Build history of the part. All positions in model axes, mm. A direction names the side the tool comes from. Round coordinates to 2 decimals unless told otherwise and drop trailing zeros. Loops run counter-clockwise (first coordinate to the right, second up) from the corner with the lowest first, then second, coordinate; pieces in that order, holes last. Notation, with made-up numbers: M 58.25,26.25 L 83.25,26.25 A18 cw 83.25,36.25 Z; hole C 32,54.5 d5. An arc over 180 degrees is marked long. Write each question's results on one line, items separated by ' | '. Start each with the question number.
```python
from build123d import *

# Parameters (mm, degrees)
SKETCH1_W           = 30
SKETCH1_H           = 30
BOSS_EXTRUDE2_DEPTH = 15
SKETCH3_W           = 20
SKETCH3_H           = 20
CUT_EXTRUDE1_DEPTH  = 5
SKETCH4_R           = 5
CUT_EXTRUDE2_DEPTH  = 8
SKETCH7_R           = 2
CUT_EXTRUDE4_DEPTH  = 25
SKETCH8_W           = 10
SKETCH8_H           = 10
CUT_EXTRUDE7_DEPTH  = 25
SKETCH9_W           = 30
SKETCH9_H           = 8
CUT_EXTRUDE8_DEPTH  = 25
FILLET1_R           = 2
FILLET2_R           = 2


with BuildPart() as part:
    # Sketch1 → Boss-Extrude2 (new body)
    with BuildSketch(Plane(origin=(0, 0, 0), x_dir=(1, 0, 0), z_dir=(0, 1, 0))):
        with Locations((15, 15)):
            Rectangle(SKETCH1_W, SKETCH1_H)
    extrude(amount=BOSS_EXTRUDE2_DEPTH)

    # Sketch3 → Cut-Extrude1 (cut)
    with BuildSketch(Plane(origin=(0, 15, 0), x_dir=(1, 0, 0), z_dir=(0, 1, 0))):
        with Locations((15, 10)):
            Rectangle(SKETCH3_W, SKETCH3_H)
    extrude(amount=-CUT_EXTRUDE1_DEPTH, mode=Mode.SUBTRACT)

    # Sketch4 → Cut-Extrude2 (cut)
    with BuildSketch(Plane.XZ):
        with Locations(Location((15, -11, 0), (0, 0, 270))):
            Circle(SKETCH4_R)
    extrude(amount=-CUT_EXTRUDE2_DEPTH, mode=Mode.SUBTRACT)

    # Sketch7 → Cut-Extrude4 (cut)
    with BuildSketch(Plane(origin=(0, 10, 0), x_dir=(1, 0, 0), z_dir=(0, 1, 0))):
        with Locations(Location((7, 18, 0), (0, 0, 90))):
            Circle(SKETCH7_R)
        with Locations(Location((23, 18, 0), (0, 0, 90))):
            Circle(SKETCH7_R)
    extrude(amount=-CUT_EXTRUDE4_DEPTH, mode=Mode.SUBTRACT)

    # Sketch8 → Cut-Extrude7 (cut)
    with BuildSketch(Plane(origin=(0, 15, 0), x_dir=(1, 0, 0), z_dir=(0, 1, 0))):
        with Locations((15, 25)):
            Rectangle(SKETCH8_W, SKETCH8_H)
    extrude(amount=-CUT_EXTRUDE7_DEPTH, mode=Mode.SUBTRACT)

    # Sketch9 → Cut-Extrude8 (cut)
    with BuildSketch(Plane(origin=(0, 15, 0), x_dir=(1, 0, 0), z_dir=(0, 1, 0))):
        with Locations((15, 26)):
            Rectangle(SKETCH9_W, SKETCH9_H)
    extrude(amount=-CUT_EXTRUDE8_DEPTH, mode=Mode.SUBTRACT)

    # Fillet1
    # the kernel refuses this fillet: 2 mm, written as the material it takes off along each edge
    with BuildSketch(Plane(origin=(20, 0, -20), x_dir=(1, 0, 0), z_dir=(0, 0, -1)), Plane(origin=(10, 0, -27), x_dir=(-1, 0, 0), z_dir=(0, 0, 1))) as fillet1_piece_1:
        with BuildLine():
            CenterArc((FILLET1_R, -FILLET1_R), FILLET1_R, 90, 90)
            Line((0, -FILLET1_R), (0, 0))
            Line((0, 0), (FILLET1_R, 0))
        make_face()
    extrude(amount=7, mode=Mode.SUBTRACT)
    with BuildSketch(Plane(origin=(10, 0, -20), x_dir=(0, 0, 1), z_dir=(1, 0, 0))) as fillet1_piece_2:
        with BuildLine():
            CenterArc((FILLET1_R, -FILLET1_R), FILLET1_R, 90, 90)
            Line((0, -FILLET1_R), (0, 0))
            Line((0, 0), (FILLET1_R, 0))
        make_face()
    extrude(amount=10, mode=Mode.SUBTRACT)
    with BuildSketch(Plane(origin=(15, 0, -22), x_dir=(0, 0, 1), z_dir=(-1, 0, 0)), Plane(origin=(35, 0, -22), x_dir=(0, 0, 1), z_dir=(-1, 0, 0))) as fillet1_piece_3:
        with BuildLine():
            CenterArc((FILLET1_R, FILLET1_R), FILLET1_R, 180, 90)
            Line((0, FILLET1_R), (0, 0))
            Line((0, 0), (FILLET1_R, 0))
        make_face()
    extrude(amount=20, mode=Mode.SUBTRACT)
    with BuildSketch(Plane(origin=(0, 0, -27), x_dir=(1, 0, 0), z_dir=(0, 0, 1)), Plane(origin=(30, 0, 5), x_dir=(-1, 0, 0), z_dir=(0, 0, -1))) as fillet1_piece_4:
        with BuildLine():
            CenterArc((FILLET1_R, FILLET1_R), FILLET1_R, 180, 90)
            Line((0, FILLET1_R), (0, 0))
            Line((0, 0), (FILLET1_R, 0))
        make_face()
    extrude(amount=32, mode=Mode.SUBTRACT)
    with BuildSketch(Plane(origin=(-5, 0, 0), x_dir=(0, 1, 0), z_dir=(1, 0, 0))) as fillet1_piece_5:
        with BuildLine():
            CenterArc((FILLET1_R, -FILLET1_R), FILLET1_R, 90, 90)
            Line((0, -FILLET1_R), (0, 0))
            Line((0, 0), (FILLET1_R, 0))
        make_face()
    extrude(amount=40, mode=Mode.SUBTRACT)
    with BuildSketch(Plane(origin=(10, 0, -20), x_dir=(0, 0, 1), z_dir=(1, 0, 0))) as fillet1_piece_6a_section:
        with BuildLine():
            CenterArc((FILLET1_R, -FILLET1_R), FILLET1_R, 90, 90)
            Line((0, -FILLET1_R), (0, 0))
            Line((0, 0), (FILLET1_R, 0))
        make_face()
    fillet1_piece_6a = extrude(amount=15, mode=Mode.PRIVATE)
    fillet1_piece_6a = split(fillet1_piece_6a, bisect_by=Plane(origin=(20, 0.452790229, -19.547209771), z_dir=(1, 0, 0)), keep=Keep.TOP, mode=Mode.PRIVATE)
    with BuildSketch(Plane(origin=(20, 0, -15), x_dir=(1, 0, 0), z_dir=(0, 0, -1))) as fillet1_piece_6b_section:
        with BuildLine():
            CenterArc((FILLET1_R, -FILLET1_R), FILLET1_R, 90, 90)
            Line((0, -FILLET1_R), (0, 0))
            Line((0, 0), (FILLET1_R, 0))
        make_face()
    fillet1_piece_6b = extrude(amount=12, mode=Mode.PRIVATE)
    fillet1_piece_6b = split(fillet1_piece_6b, bisect_by=Plane(origin=(20.452790229, 0.452790229, -20), z_dir=(0, 0, 1)), keep=Keep.TOP, mode=Mode.PRIVATE)
    fillet1_piece_6 = fillet1_piece_6a & fillet1_piece_6b
    add(fillet1_piece_6, mode=Mode.SUBTRACT)
    with BuildSketch(Plane(origin=(10, 0, -27), x_dir=(-1, 0, 0), z_dir=(0, 0, 1))) as fillet1_piece_7a_section:
        with BuildLine():
            CenterArc((FILLET1_R, -FILLET1_R), FILLET1_R, 90, 90)
            Line((0, -FILLET1_R), (0, 0))
            Line((0, 0), (FILLET1_R, 0))
        make_face()
    fillet1_piece_7a = extrude(amount=12, mode=Mode.PRIVATE)
    fillet1_piece_7a = split(fillet1_piece_7a, bisect_by=Plane(origin=(9.547209771, 0.452790229, -20), z_dir=(0, 0, 1)), keep=Keep.TOP, mode=Mode.PRIVATE)
    with BuildSketch(Plane(origin=(5, 0, -20), x_dir=(0, 0, 1), z_dir=(1, 0, 0))) as fillet1_piece_7b_section:
        with BuildLine():
            CenterArc((FILLET1_R, -FILLET1_R), FILLET1_R, 90, 90)
            Line((0, -FILLET1_R), (0, 0))
            Line((0, 0), (FILLET1_R, 0))
        make_face()
    fillet1_piece_7b = extrude(amount=15, mode=Mode.PRIVATE)
    fillet1_piece_7b = split(fillet1_piece_7b, bisect_by=Plane(origin=(10, 0.452790229, -19.547209771), z_dir=(-1, 0, 0)), keep=Keep.TOP, mode=Mode.PRIVATE)
    fillet1_piece_7 = fillet1_piece_7a & fillet1_piece_7b
    add(fillet1_piece_7, mode=Mode.SUBTRACT)

    # Fillet2
    # the kernel refuses this fillet: 2 mm, written as the material it takes off along each edge
    with BuildSketch(Plane(origin=(2, 2, -2), x_dir=(-1, 0, 0), z_dir=(0, 0, 1))) as fillet2_piece_1_section:
        Polygon((0, 0), (FILLET2_R, 0), (FILLET2_R, FILLET2_R), (0, FILLET2_R), align=None)
    fillet2_piece_1 = extrude(amount=FILLET2_R, mode=Mode.PRIVATE)
    fillet2_piece_1 = fillet2_piece_1 - Plane(origin=(2, 2, -2), x_dir=(0.7071067811865475, 0.7071067811865475, 0), z_dir=(0, 0, 1)) * Sphere(FILLET2_R, mode=Mode.PRIVATE)
    add(fillet2_piece_1, mode=Mode.SUBTRACT)
    with BuildSketch(Plane(origin=(2, 2, -20), x_dir=(0, 0, -1), z_dir=(-1, 0, 0))) as fillet2_piece_2_section:
        Polygon((0, 0), (FILLET2_R, 0), (FILLET2_R, FILLET2_R), (0, FILLET2_R), align=None)
    fillet2_piece_2 = extrude(amount=FILLET2_R, mode=Mode.PRIVATE)
    fillet2_piece_2 = fillet2_piece_2 - Plane(origin=(2, 2, -20), x_dir=(0, 0.7071067811865475, 0.7071067811865475), z_dir=(-1, 0, 0)) * Sphere(FILLET2_R, mode=Mode.PRIVATE)
    add(fillet2_piece_2, mode=Mode.SUBTRACT)
    with BuildSketch(Plane(origin=(8, 2, -20), x_dir=(1, 0, 0), z_dir=(0, 0, -1))) as fillet2_piece_3_section:
        Polygon((0, 0), (FILLET2_R, 0), (FILLET2_R, FILLET2_R), (0, FILLET2_R), align=None)
    fillet2_piece_3 = extrude(amount=FILLET2_R, mode=Mode.PRIVATE)
    fillet2_piece_3 = fillet2_piece_3 - Plane(origin=(8, 2, -20), x_dir=(-0.7071067811865475, 0.7071067811865475, 0), z_dir=(0, 0, -1)) * Sphere(FILLET2_R, mode=Mode.PRIVATE)
    add(fillet2_piece_3, mode=Mode.SUBTRACT)
    with BuildSketch(Plane(origin=(28, 2, -2), x_dir=(1, 0, 0), z_dir=(0, 0, 1))) as fillet2_piece_4_section:
        Polygon((0, 0), (FILLET2_R, 0), (FILLET2_R, -FILLET2_R), (0, -FILLET2_R), align=None)
    fillet2_piece_4 = extrude(amount=FILLET2_R, mode=Mode.PRIVATE)
    fillet2_piece_4 = fillet2_piece_4 - Plane(origin=(28, 2, -2), x_dir=(-0.7071067811865475, 0.7071067811865475, 0), z_dir=(0, 0, 1)) * Sphere(FILLET2_R, mode=Mode.PRIVATE)
    add(fillet2_piece_4, mode=Mode.SUBTRACT)
    with BuildSketch(Plane(origin=(22, 2, -20), x_dir=(0, 0, -1), z_dir=(-1, 0, 0))) as fillet2_piece_5_section:
        Polygon((0, 0), (FILLET2_R, 0), (FILLET2_R, FILLET2_R), (0, FILLET2_R), align=None)
    fillet2_piece_5 = extrude(amount=FILLET2_R, mode=Mode.PRIVATE)
    fillet2_piece_5 = fillet2_piece_5 - Plane(origin=(22, 2, -20), x_dir=(0, 0.7071067811865475, 0.7071067811865475), z_dir=(-1, 0, 0)) * Sphere(FILLET2_R, mode=Mode.PRIVATE)
    add(fillet2_piece_5, mode=Mode.SUBTRACT)
    with BuildSketch(Plane(origin=(28, 2, -20), x_dir=(1, 0, 0), z_dir=(0, 0, -1))) as fillet2_piece_6_section:
        Polygon((0, 0), (FILLET2_R, 0), (FILLET2_R, FILLET2_R), (0, FILLET2_R), align=None)
    fillet2_piece_6 = extrude(amount=FILLET2_R, mode=Mode.PRIVATE)
    fillet2_piece_6 = fillet2_piece_6 - Plane(origin=(28, 2, -20), x_dir=(-0.7071067811865475, 0.7071067811865475, 0), z_dir=(0, 0, -1)) * Sphere(FILLET2_R, mode=Mode.PRIVATE)
    add(fillet2_piece_6, mode=Mode.SUBTRACT)
    with BuildSketch(Plane(origin=(2, 13, -20), x_dir=(0, 0, -1), z_dir=(-1, 0, 0))) as fillet2_piece_7_section:
        Polygon((0, 0), (FILLET2_R, 0), (FILLET2_R, -FILLET2_R), (0, -FILLET2_R), align=None)
    fillet2_piece_7 = extrude(amount=FILLET2_R, mode=Mode.PRIVATE)
    fillet2_piece_7 = fillet2_piece_7 - Plane(origin=(2, 13, -20), x_dir=(0, -0.7071067811865475, 0.7071067811865475), z_dir=(-1, 0, 0)) * Sphere(FILLET2_R, mode=Mode.PRIVATE)
    add(fillet2_piece_7, mode=Mode.SUBTRACT)
    with BuildSketch(Plane(origin=(28, 13, -20), x_dir=(1, 0, 0), z_dir=(0, 1, 0))) as fillet2_piece_8_section:
        Polygon((0, 0), (FILLET2_R, 0), (FILLET2_R, FILLET2_R), (0, FILLET2_R), align=None)
    fillet2_piece_8 = extrude(amount=FILLET2_R, mode=Mode.PRIVATE)
    fillet2_piece_8 = fillet2_piece_8 - Plane(origin=(28, 13, -20), x_dir=(-0.7071067811865475, 0, 0.7071067811865475), z_dir=(0, 1, 0)) * Sphere(FILLET2_R, mode=Mode.PRIVATE)
    add(fillet2_piece_8, mode=Mode.SUBTRACT)
    with BuildSketch(Plane(origin=(0, 15, -20), x_dir=(0, -1, 0), z_dir=(0, 0, 1))) as fillet2_piece_9:
        with BuildLine():
            CenterArc((FILLET2_R, FILLET2_R), FILLET2_R, 180, 90)
            Line((0, FILLET2_R), (0, 0))
            Line((0, 0), (FILLET2_R, 0))
        make_face()
    extrude(amount=25, mode=Mode.SUBTRACT)
    with BuildSketch(Plane(origin=(0, 2, 0), x_dir=(1, 0, 0), z_dir=(0, 1, 0)), Plane(origin=(20, 2, -22), x_dir=(0, 0, 1), z_dir=(0, 1, 0))) as fillet2_piece_10:
        with BuildLine():
            CenterArc((FILLET2_R, FILLET2_R), FILLET2_R, 180, 90)
            Line((0, FILLET2_R), (0, 0))
            Line((0, 0), (FILLET2_R, 0))
        make_face()
    extrude(amount=18, mode=Mode.SUBTRACT)
    with BuildSketch(Plane(origin=(15, 15, -22), x_dir=(0, -1, 0), z_dir=(-1, 0, 0)), Plane(origin=(28, 15, -22), x_dir=(0, -1, 0), z_dir=(-1, 0, 0))) as fillet2_piece_11:
        with BuildLine():
            CenterArc((FILLET2_R, FILLET2_R), FILLET2_R, 180, 90)
            Line((0, FILLET2_R), (0, 0))
            Line((0, 0), (FILLET2_R, 0))
        make_face()
    extrude(amount=13, mode=Mode.SUBTRACT)
    with BuildSketch(Plane(origin=(0, 13, -22), x_dir=(0, 0, 1), z_dir=(0, -1, 0)), Plane(origin=(30, 13, -22), x_dir=(-1, 0, 0), z_dir=(0, -1, 0))) as fillet2_piece_12:
        with BuildLine():
            CenterArc((FILLET2_R, -FILLET2_R), FILLET2_R, 90, 90)
            Line((0, -FILLET2_R), (0, 0))
            Line((0, 0), (FILLET2_R, 0))
        make_face()
    extrude(amount=11, mode=Mode.SUBTRACT)
    with BuildSketch(Plane(origin=(10, 20, -22), x_dir=(-1, 0, 0), z_dir=(0, -1, 0)), Plane(origin=(30, 2, 0), x_dir=(-1, 0, 0), z_dir=(0, 1, 0))) as fillet2_piece_13:
        with BuildLine():
            CenterArc((FILLET2_R, -FILLET2_R), FILLET2_R, 90, 90)
            Line((0, -FILLET2_R), (0, 0))
            Line((0, 0), (FILLET2_R, 0))
        make_face()
    extrude(amount=18, mode=Mode.SUBTRACT)
    with BuildSketch(Plane(origin=(30, 15, 5), x_dir=(-1, 0, 0), z_dir=(0, 0, -1))) as fillet2_piece_14:
        with BuildLine():
            CenterArc((FILLET2_R, -FILLET2_R), FILLET2_R, 90, 90)
            Line((0, -FILLET2_R), (0, 0))
            Line((0, 0), (FILLET2_R, 0))
        make_face()
    extrude(amount=25, mode=Mode.SUBTRACT)


solid = part.part
```
Item 1: Tool access for faces 5 (the cylindrical face through (20.6, 8.41, -21.43)), 6 (the cylindrical face through (10.564, 3.944, -13.307)), 7 (the flat face through (5, 13, -10)), 8 (the cylindrical face through (9.13, 0.35, -19.68)): list every direction of +Z, -Z, +X, -X, +Y, -Y with a clear straight run to the whole face (end or side of a thin tool).
Item 2: Drop flat-ended pins along their axis: pin 1 (4 mm diameter, centred on x = 21.5, y = 12.5, fed in from +Z); pin 2 (2 mm diameter, centred on x = 12, z = -9, fed in from -Y); pin 3 (9 mm diameter, centred on x = 15, z = -11, fed in from +Y). Give the stop position or say it passes through.
Item 3: Mould opens along X. For faces 1 (the cylindrical face through (29.4, 14.43, -9.86)), 2 (the cylindrical face through (14.91, 0.57, -19.4)), 3 (the cylindrical face through (9.4, 8.59, -21.43)), 4 (the flat face through (25, 8, -22)) say: released by +X, released by -X, zero draft, split by the parting line, or undercut.
Item 4: Saw through at D-D, the plane x = 15. Give the cut face in (y, z).
Item 5: Saw through at B-B, the plane y = 6.25. Give the cut face in (x, z), then the cut area to 3 significant figures.
Item 6: Saw through at C-C, the plane z = -2.5. Give the cut face in (x, y), then the cut area to 3 significant figures.
Item 7: Saw through at A-A, the plane y = 12.25. Give the cut face in (x, z).
Item 8: Drill centre lines: line 1 along X through (y, z) = (8.25, -18); line 2 along X through (y, z) = (3.25, -11); line 3 along Z through (x, y) = (7, 7.25). Where is each one in solid material? Low to high. Write a range as [from, to].
Working result:
1) face 5: -Z, +Y, -Y | face 6: -Y | face 7: +Z, +Y | face 8: -Z, -Y
2) pin 1: stops at z = -20 | pin 2: stops at y = 8 | pin 3: stops at y = 10
3) face 1: released by +X | face 2: undercut | face 3: undercut | face 4: zero draft
4) outline: M 0,-18 A2 ccw 2,-20 L 10,-20 L 10,0 L 2,0 A2 ccw 0,-2 L 0,-6 L 8,-6 L 8,-16 L 0,-16 Z
5) outline: M 0,-20 A2 ccw 2,-22 L 8,-22 A2 ccw 10,-20 L 20,-20 A2 ccw 22,-22 L 28,-22 A2 ccw 30,-20 L 30,-2 A2 ccw 28,0 L 2,0 A2 ccw 0,-2 Z; hole C 7,-18 d4; hole C 15,-11 d10; hole C 23,-18 d4 | area: 531 mm²
6) outline: M 0,2 A2 ccw 2,0 L 28,0 A2 ccw 30,2 L 30,13 A2 ccw 28,15 L 25,15 L 25,10 L 5,10 L 5,15 L 2,15 A2 ccw 0,13 Z | area: 347 mm²
7) outline: M 0,-20 A2 ccw 2,-22 L 8,-22 A2 ccw 10,-20 L 5,-20 L 5,0 L 2,0 A2 ccw 0,-2 Z; M 20,-20 A2 ccw 22,-22 L 28,-22 A2 ccw 30,-20 L 30,-2 A2 ccw 28,0 L 25,0 L 25,-20 Z
8) line 1: x = [0, 5], [9, 21], [25, 30] | line 2: x = [0, 10], [20, 30] | line 3: z = [-22, -20], [-16, 0]
